Part model, mm, in its own coordinate system. A direction names the side the tool comes from. Coordinates: 2 decimals unless noted, no trailing zeros. Loops run counter-clockwise (first coordinate to the right, second up) from the corner with the lowest first, then second, coordinate; pieces in that order, holes last. Notation, with made-up numbers: M -20,69.25 L -7,69.25 A21 cw -7,97.25 Z; hole C 57.5,52 d6. An arc over 180 degrees is marked long. Answer as a JSON object with one key per item and string values. Group by question number.
1. Saw through at D-D on x = 0. Write the cut outline in (y, z).
2. Saw through at C-C on z = 10.5. Write the cut outline in (x, y).
3. Saw through at A-A on y = -15.5. Write the cut outline in (x, z).
4. Mould opens along Y. For faces 1 (the face through (-20, 20, 16)), 2 (the face through (0, 0, -1.5)), 3 (the face through (14, 15.57, 16.73)) say: released by +Y, released by -Y, zero draft, split by the parting line, or undercut.
5. Drill centre lines: L1, parallel to Y at x = 15.5, z = 15; L2, parallel to Y at x = -15, z = 13. Where is each one in solid material? Low to high.
6. 3-axis set-ups, long thin cutter, end or side, ignore diameter. For faces 4 (the face through (-5.525, -3.131, 38.712)), 5 (the face through (-0.54, -2.44, -0.76)), 6 (the face through (5.525, 3.131, 38.712)), 7 (the face through (-0.54, -2.44, 45.69)), 8 (the face through (0, -6.35, 39)): which of +Z, -Z, +X, -X, +Y, -Y reach the whole face in a straight line?
7. Drop flat-ended pins along their axis: pin 1 Ø4 at (y, z) = (6.5, 38.5) entering from +X; pin 2 Ø5 at (x, y) = (15.5, 15.5) entering from +Z; pin 3 Ø1.6 at (x, z) = (1, 39) entering from -Y; pin 4 Ø10 at (x, y) = (2.5, 0.5) entering from -Z. Give the stop position or say it passes through.
from build123d import *

# Parameters (mm, degrees)
EXTRUDE1_DEPTH      = 33
SKETCH2_R           = 1.5
EXTRUDE2_DEPTH      = 43
SKETCH3_R           = 11
EXTRUDE3_DEPTH      = 2.5
EXTRUDE4_DEPTH      = 14.5
EXTRUDE4_DEPTH_BACK = 37
SKETCH4_R           = 2.5
BOSS_EXTRUDE1_START = 0.5
BOSS_EXTRUDE1_DEPTH = 5.5


with BuildPart() as part:
    # Sketch1 → Extrude1 (new body)
    with BuildSketch(Plane.XY):
        Polygon((-21, 19), (-19, 21), (19, 21), (21, 19), (21, -19), (19, -21), (-19, -21), (-21, -19), align=None)
    extrude(amount=EXTRUDE1_DEPTH)

    # Sketch2 → Extrude2 (cut)
    with BuildSketch(Plane.XY.offset(33)):
        with Locations((-15.5, 15.5)):
            Circle(SKETCH2_R)
        with Locations((15.5, 15.5)):
            Circle(SKETCH2_R)
        with Locations((-15.5, -15.5)):
            Circle(SKETCH2_R)
        with Locations((15.5, -15.5)):
            Circle(SKETCH2_R)
    extrude(amount=-EXTRUDE2_DEPTH, mode=Mode.SUBTRACT)

    # Sketch3 → Extrude3 (add)
    with BuildSketch(Plane.XY.offset(33)):
        with Locations(Location((0, 0, 0), (0, 0, 180))):
            Circle(SKETCH3_R)
    extrude(amount=EXTRUDE3_DEPTH)

    # Sketch4 → Extrude4 (add, two sides: drawn at the far end of the back side and taken through both)
    with BuildSketch(Plane.XY.offset(35.5).offset(-EXTRUDE4_DEPTH_BACK)):
        Circle(SKETCH4_R)
    extrude(amount=EXTRUDE4_DEPTH + EXTRUDE4_DEPTH_BACK)

    # Sketch5 → Boss-Extrude1 (add)
    with BuildSketch(Plane.XY.offset(35.5).offset(BOSS_EXTRUDE1_START)):
        Polygon((7.332348419, 0), (3.666174209, 6.35), (-3.666174209, 6.35), (-7.332348419, 0), (-3.666174209, -6.35), (3.666174209, -6.35), align=None)
    extrude(amount=BOSS_EXTRUDE1_DEPTH)


solid = part.part
Outcome:
{
 "1": {"outline": "M -21,0 L -2.5,0 L -2.5,-1.5 L 2.5,-1.5 L 2.5,0 L 21,0 L 21,33 L 11,33 L 11,35.5 L 2.5,35.5 L 2.5,36 L 6.35,36 L 6.35,41.5 L 2.5,41.5 L 2.5,50 L -2.5,50 L -2.5,41.5 L -6.35,41.5 L -6.35,36 L -2.5,36 L -2.5,35.5 L -11,35.5 L -11,33 L -21,33 Z"},
 "2": {"outline": "M -21,-19 L -19,-21 L 19,-21 L 21,-19 L 21,19 L 19,21 L -19,21 L -21,19 Z; hole C -15.5,-15.5 d3; hole C -15.5,15.5 d3; hole C 15.5,-15.5 d3; hole C 15.5,15.5 d3"},
 "3": {"outline": "M -21,0 L -17,0 L -17,33 L -21,33 Z; M -14,0 L 14,0 L 14,33 L -14,33 Z; M 17,0 L 21,0 L 21,33 L 17,33 Z"},
 "4": {"face 1": "released by +Y", "face 2": "zero draft", "face 3": "undercut"},
 "5": {"L1": "y = -21 to -17, -14 to 14, 17 to 21", "L2": "y = -21 to -16.91, -14.09 to 14.09, 16.91 to 21"},
 "6": {"face 4": "+Z, -X, -Y", "face 5": "-Z", "face 6": "+Z, +X, +Y", "face 7": "+Z", "face 8": "+Z, +X, -X, -Y"},
 "7": {"pin 1": "stops at x = 4.73", "pin 2": "stops at z = 33", "pin 3": "stops at y = -6.35", "pin 4": "stops at z = -1.5"}
}
